Autodesk Inventor part; units mm, degrees
ref_plane "YZ Plane" through (0, 0, 0) normal (1, 0, 0) x (0, 1, 0)
ref_plane "XZ Plane" through (0, 0, 0) normal (0, 1, 0) x (-1, 0, 0)
ref_plane "XY Plane" through (0, 0, 0) normal (0, 0, 1) x (1, 0, 0)
sketch "Sketch1" plane through (0, 0, 0) normal (0, 0, 1) x (1, 0, 0)
  line L0 (0, 0) -> (0, 38.4841) construction
  line L1 (2.8, 19) -> (3.8, 18)
  line L2 (3.8, 18) -> (3.8, 0)
  line L3 (2.8, 19) -> (1.4, 19)
  line L4 (1.4, 19) -> (1.4, 0)
  line L5 (1.4, 0) -> (3.8, 0)
  dimension "d1" = 1.4
  dimension "d8" = 1
  dimension "d20" = 3.8
  dimension "d46" = 19
revolve "Revolution1" add sketch "Sketch1" angle 360 about axis through (0, 0, 0) along (0, 1, 0)
chamfer "Chamfer1" distance 0.5 angle 45 2 edges at (-1.4, 19, 0) (-1.4, 0, 0)
sketch "Sketch6" plane through (0, 0, 0) normal (0, -1, 0) x (1, 0, 0)
  line L0 (0, 0) -> (0, -8) construction
  circle A0 centre (0, 8) radius 3
  circle A1 centre (0, -8) radius 3
  circle A2 centre (0, 0) radius 6
  line L1 (0, 0) -> (0, 8) construction
  circle A3 centre (0, 8) radius 1.35
  circle A4 centre (0, -8) radius 1.35
  circle A5 centre (0, 0) radius 1.9
  line L2 (11.8, 4.2) -> (2, 4.2)
  line L3 (2, 4.2) -> (2, -4.2)
  line L4 (2, -4.2) -> (11.8, -4.2)
  line L5 (11.8, -4.2) -> (11.8, 4.2)
  line L6 (0, 0) -> (2, 4.2) construction
  line L7 (0, 0) -> (2, -4.2) construction
  point P0 (1.9111, -5.6875)
  point P1 (1.9111, 5.6875)
  point P2 (-1.9111, 5.6875)
  point P3 (-1.9111, -5.6875)
  point P4 (4.2849, 4.2)
  point P5 (4.2849, -4.2)
  dimension "d24" = 6
  dimension "d26" = 8
  dimension "d27" = 12
  dimension "d28" = 2.7
  dimension "d33" = 2
  dimension "d34" = 8.4
  dimension "d35" = 11.8
extrude "Extrusion3" add sketch "Sketch6" against normal blind 14.2
fillet "Fillet1" radius 4 4 edges at (-1.9111, 7.1, 5.6875) (1.9111, 7.1, 5.6875) (1.9111, 7.1, -5.6875) (-1.9111, 7.1, -5.6875)
sketch "Sketch7" plane through (0, 0, -8) normal (0, -1, 0) x (1, 0, 0)
  circle A0 centre (0, 8) radius 6
sketch "Sketch8" plane through (0, 0, 8) normal (0, -1, 0) x (1, 0, 0)
  point P0 (0, -8)
sketch "Sketch10" plane through (11.8, 0, 4.2) normal (1, 0, 0) x (0, 0, -1)
  line L0 (7.2, 1.2) -> (1.2, 1.2)
  line L1 (1.2, 1.2) -> (1.2, 14.2)
  line L2 (1.2, 14.2) -> (7.2, 14.2)
  line L3 (7.2, 14.2) -> (7.2, 1.2)
  line L4 (7.2, 1.2) -> (4.2, 0) construction
  line L5 (4.2, 0) -> (1.2, 1.2) construction
  line L6 (8.4, 0) -> (0, 0)
  dimension "d39" = 6
  dimension "d40" = 1.2
  dimension "d41" = 13
extrude "Extrusion4" cut sketch "Sketch10" against normal blind 8
fillet "Fillet4" radius 3 2 edges at (4.2849, 7.1, 4.2) (4.2849, 7.1, -4.2)
fillet "Fillet5" radius 0.5 7 edges at (2.961, 14.2, -7.446) (-6, 14.2, 0) (2.961, 14.2, 7.446) (0, 14.2, 11) (8.8764, 14.2, 4.2) (8.8764, 14.2, -4.2) (0, 14.2, -11)
properties part number "caster-bng"
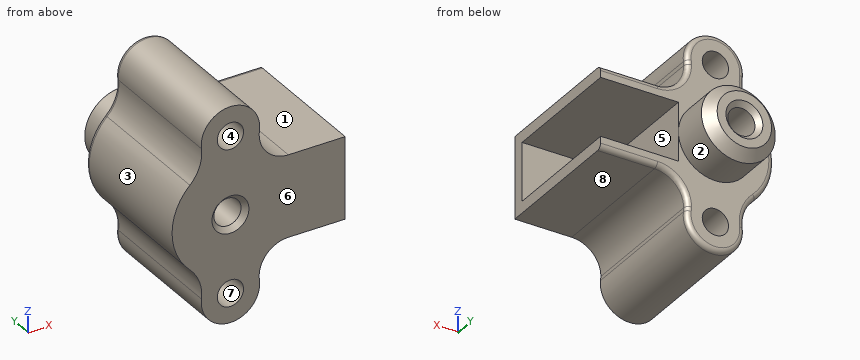
The model under review builds one solid part; all positions refer to its coordinate system, in mm. Face numbers are marked on the shaded views. A direction names the side the tool comes from. Round coordinates to 2 decimals unless told otherwise and drop trailing zeros. Order: outer loops, then holes, each group sorted by start corner. A loop starts at its lowest first (then second) coordinate and runs counter-clockwise, first axis right, second up. Notation, with made-up numbers: (88, 83) - (113, 83) arc R29 ccw to (113, 113) - close; hole circle Ø10 at (66, 55). An arc over 180 degrees is marked (long way). Answer in a Markdown table with one row per item.
(1) For line 1 (Z direction, x = 0, y = 4.5); line 2 (Z direction, x = 6, y = 9.25); line 3 (Z direction, x = -0.75, y = 4.75), list the stretches that pass through material, from the lowest coordinate up. Write a range as from..to.
Result set:
| item | result |
|---|---|
| line 1 | z = -11..-9.35, -6.65..-1.4, 1.4..6.65, 9.35..11 |
| line 2 | z = -4.2..-3, 3..4.2 |
| line 3 | z = -10.9..-9.12, -6.88..-1.18, 1.18..6.88, 9.12..10.9 |
(2) Mouldability with a two-part tool opening along Z and no side actions: class the marked faces 6, 7 and 8 as released by +Z, released by -Z, zero draft, split by the parting line, or undercut.
Result set:
| item | result |
|---|---|
| face 6 | zero draft |
| face 7 | undercut |
| face 8 | released by -Z |
(3) Take a section at C-C on y = 17. Write out the cut boundary in (x, z), plus the area to 3 significant figures.
Result set:
| item | result |
|---|---|
| outline | circle Ø7.6 at (0, 0); hole circle Ø2.8 at (0, 0) |
| area | 39.2 mm2 |
(4) Take a section at A-A on z = -8. Write out the cut boundary in (x, y), plus the area to 3 significant figures.
Result set:
| item | result |
|---|---|
| outline | (-3, 0) - (-1.35, 0) - (-1.35, 14.2) - (-2.5, 14.2) arc R0.5 ccw to (-3, 13.7) - close; (1.35, 0) - (3, 0) - (3, 13.7) arc R0.5 ccw to (2.5, 14.2) - (1.35, 14.2) - close |
| area | 46.8 mm2 |
(5) Clearance check with flat-ended pins moving along their axes: P1, Ø6, axis at x = 2, z = -2.5, coming from the +Y side; P2, Ø3, axis at x = 7.5, z = 1, coming from the +Y side; P3, Ø2, axis at y = 13.5, z = -5, coming from the -X side; P4, Ø3, axis at x = 0, z = -8, coming from the +Y side. State where each tip first meets the part, or that it passes through.
Result set:
| item | result |
|---|---|
| P1 | stops at y = 19 |
| P2 | stops at y = 1.2 |
| P3 | stops at x = -4.47 |
| P4 | stops at y = 14.2 |
(6) Take a section at B-B on x = 7.5. Write out the cut boundary in (y, z), plus the area to 3 significant figures.
Result set:
| item | result |
|---|---|
| outline | (0, -4.2) - (13.7, -4.2) arc R0.5 ccw to (14.2, -3.7) - (14.2, -3) - (1.2, -3) - (1.2, 3) - (14.2, 3) - (14.2, 3.7) arc R0.5 ccw to (13.7, 4.2) - (0, 4.2) - close |
| area | 41.2 mm2 |
(7) Machinability: for the marked faces 1, 2, 3, 4 and 5, which of the approach directions +Z, -Z, +X, -X, +Y, -Y give a long, thin tool a straight path to every point of the face, cutting with its end or side? Answer none if there is none.
Result set:
| item | result |
|---|---|
| face 1 | +Z, +X, +Y, -Y |
| face 2 | +Y |
| face 3 | -X, +Y, -Y |
| face 4 | +Y, -Y |
| face 5 | +X, +Y |
(8) Take a section at D-D on y = 12.75. Count the separate pieces of the cut face and the enclosed holes in it, plus the area to 3 significant figures.
Result set:
| item | result |
|---|---|
| separate pieces | 1 |
| enclosed holes | 3 |
| area | 159 mm2 |
